Work out the finished part from the listing and answer in its coordinate system (mm). Coordinates: 2 decimals unless noted, no trailing zeros. Write each loop counter-clockwise with the first axis right and the second up, starting at its lowest first coordinate (ties: lowest second). Pieces come first, ordered by that corner, then holes. Notation, with made-up numbers: M -3,54 L 12,54 A23 ccw 12,81 Z; hole C 13.5,-25 d6. An arc over 180 degrees is marked long. Answer as CSV lines item,"result". Start each with the question number.
(1) Flat-ended cylindrical pins translate along their axes: P1, Ø0.6, axis at x = 35, y = 1, coming from the +Z side; P2, Ø1, axis at y = 1.5, z = -20, coming from the +X side; P3, Ø0.6, axis at x = 5, y = 1.5, coming from the +Z side. Find the tip coordinate at first contact, or state that the pin passes through.
(2) A cutting plane is placed at A-A on x = -13.57. Give the vertices of the cut face in (y, z).
(3) Find the intervals of material crossed by L1, parallel to Z at x = -13.57, y = 0.85; L2, parallel to X at y = 1.15, z = 2; L3, parallel to Z at x = 17.5, y = 0.85, in increasing order. Write a range as [from, to].
(4) A cutting plane is placed at C-C on z = 29. Give the vertices of the cut face in (x, y).
(5) A cutting plane is placed at B-B on z = -19.5. Give the vertices of the cut face in (x, y).
(6) A cutting plane is placed at D-D on y = 1.7. Count the separate pieces of the cut face and the enclosed holes in it, then the cut area to 3 significant figures.
Autodesk Inventor part; units mm, degrees
ref_plane "YZ Plane" through (0, 0, 0) normal (1, 0, 0) x (0, 1, 0)
ref_plane "XZ Plane" through (0, 0, 0) normal (0, 1, 0) x (-1, 0, 0)
ref_plane "XY Plane" through (0, 0, 0) normal (0, 0, 1) x (1, 0, 0)
sketch "Sketch1" plane through (0, 0, 0) normal (0, 1, 0) x (-1, 0, 0)
  line L0 (34, 37.5) -> (-34, -37.5) construction
  line L1 (-34, 37.5) -> (34, -37.5) construction
  line L2 (34, 37.5) -> (34, 25)
  line L3 (34, 25) -> (32, 25)
  line L4 (32, 25) -> (32, 12.5)
  line L5 (32, 12.5) -> (34, 12.5)
  line L6 (34, 12.5) -> (34, 0)
  line L7 (34, 0) -> (32, 0)
  line L8 (32, 0) -> (32, -12.5)
  line L9 (32, -12.5) -> (34, -12.5)
  line L10 (34, -12.5) -> (34, -25)
  line L11 (34, -25) -> (32, -25)
  line L12 (32, -25) -> (32, -37.5)
  line L13 (34, -25) -> (34, -12.5)
  line L14 (34, 0) -> (34, 12.5)
  line L15 (34, 25) -> (34, 37.5)
  line L16 (-3, -37.5) -> (-14, -37.5)
  line L17 (-14, -37.5) -> (-14, -39.5)
  line L18 (-14, -39.5) -> (-25, -39.5)
  line L19 (-25, -39.5) -> (-25, -37.5)
  line L20 (-34, -37.5) -> (-36, -37.5)
  line L21 (-36, -37.5) -> (-36, -25)
  line L22 (-36, -25) -> (-34, -25)
  line L23 (-34, -25) -> (-34, -12.5)
  line L24 (-34, -12.5) -> (-36, -12.5)
  line L25 (-36, -12.5) -> (-36, 0)
  line L26 (-36, 0) -> (-34, 0)
  line L27 (-34, 0) -> (-34, 12.5)
  line L28 (-34, 12.5) -> (-34, 8.9552)
  line L29 (-34, 12.5) -> (-36, 12.5)
  line L30 (-36, 12.5) -> (-36, 25)
  line L31 (-36, 25) -> (-34, 25)
  line L32 (-34, -37.5) -> (-25, -37.5)
  line L33 (-14, -37.5) -> (-3, -37.5)
  line L34 (-34, -12.5) -> (-34, -25)
  line L35 (-34, 35.5) -> (-34, 25)
  line L36 (-34, 12.5) -> (-34, 0)
  line L37 (34, 37.5) -> (23, 37.5)
  line L38 (23, 37.5) -> (23, 35.5)
  line L39 (23, 35.5) -> (12, 35.5)
  line L40 (12, 35.5) -> (12, 37.5)
  line L41 (12, 37.5) -> (1, 37.5)
  line L42 (1, 37.5) -> (1, 35.5)
  line L43 (1, 35.5) -> (-10, 35.5)
  line L44 (-10, 35.5) -> (-10, 37.5)
  line L45 (-10, 37.5) -> (-21, 37.5)
  line L46 (-21, 37.5) -> (-21, 35.5)
  line L47 (-21, 35.5) -> (-34, 35.5)
  line L48 (34, 37.5) -> (23, 37.5)
  line L49 (12, 37.5) -> (1, 37.5)
  line L50 (-10, 37.5) -> (-21, 37.5)
  circle A0 centre (-2.2106, -2.0043) radius 6
  circle A1 centre (13.57, -2.0043) radius 3.5
  circle A2 centre (7.6284, 10.3335) radius 3.5
  circle A3 centre (-5.7222, 13.3806) radius 3.5
  circle A4 centre (-16.4285, 4.8426) radius 3.5
  circle A5 centre (-16.4285, -8.8513) radius 3.5
  circle A6 centre (-5.7222, -17.3893) radius 3.5
  circle A7 centre (7.6284, -14.3421) radius 3.5
  line L51 (-3, -37.5) -> (-3, -39.5)
  line L52 (-3, -39.5) -> (8, -39.5)
  line L53 (8, -39.5) -> (8, -37.5)
  line L54 (8, -37.5) -> (19, -37.5)
  line L55 (19, -37.5) -> (19, -39.5)
  line L56 (19, -39.5) -> (32, -39.5)
  line L57 (32, -39.5) -> (34, -39.5)
  line L58 (34, -39.5) -> (34, -37.5)
  line L59 (32, -37.5) -> (34, -37.5)
  point P0 (0, 0)
  point P1 (0, 0)
  point P2 (8.5, -39.5)
  point P3 (-2.5, -39.5)
  dimension "d1" = 75
  dimension "d2" = 2
  dimension "d3" = 12.5
  dimension "d4" = 12.5
  dimension "d5" = 12.5
  dimension "d6" = 12.5
  dimension "d7" = 2
  dimension "d13" = 11
  dimension "d14" = 2
  dimension "d15" = 12.5
  dimension "d16" = 12.5
  dimension "d17" = 2
  dimension "d18" = 12.5
  dimension "d19" = 12.5
  dimension "d20" = 2
  dimension "d21" = 12.5
  dimension "d22" = 11
  dimension "d23" = 11
  dimension "d24" = 11
  dimension "d25" = 11
  dimension "d28" = 12
  dimension "d29" = 7
  dimension "d30" = 360
  dimension "d33" = 9
  dimension "d34" = 11
  dimension "d35" = 11
  dimension "d36" = 2
  dimension "d37" = 11
extrude "Extrusion1" add sketch "Sketch1" along normal blind 2
properties part number "KIRI"
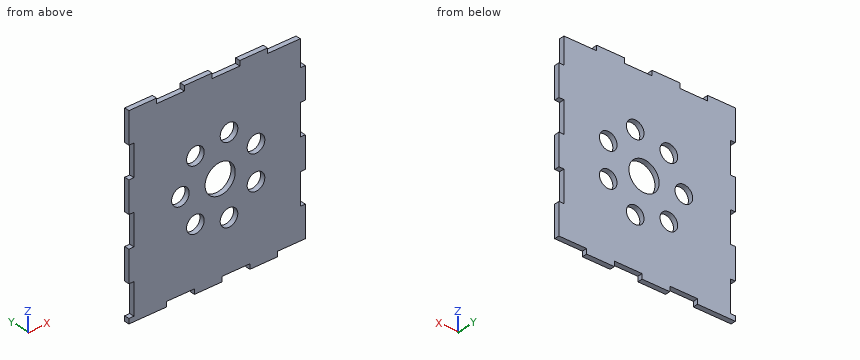
Here are the results:
1,P1,"stops at z = 25"
1,P2,"stops at x = 34"
1,P3,"stops at z = 35.5"
2,outline,"M 0,-37.5 L 2,-37.5 L 2,-5.5 L 0,-5.5 Z; M 0,1.5 L 2,1.5 L 2,35.5 L 0,35.5 Z"
3,L1,"z = [-37.5, -5.5], [1.5, 35.5]"
3,L2,"x = [-34, -2.26], [6.68, 14.39], [18.47, 34]"
3,L3,"z = [-39.5, -12.18], [-5.52, 1.51], [8.17, 37.5]"
4,outline,"M -34,0 L 34,0 L 34,2 L -34,2 Z"
5,outline,"M -34,0 L 2.93,0 L 2.93,2 L -34,2 Z; M 8.51,0 L 34,0 L 34,2 L 8.51,2 Z"
6,separate pieces,"1"
6,enclosed holes,"8"
6,area,"4,720 mm^2"
